Check sheet for the modelled part. Datum: model origin and axes. Units: mm. A direction names the side the tool comes from. Round coordinates to 2 decimals unless told otherwise and drop trailing zeros. Order: outer loops, then holes, each group sorted by start corner. A loop starts at its lowest first (then second) coordinate and runs counter-clockwise, first axis right, second up. Notation, with made-up numbers: (59, 64.5) -> (81, 64.5) arc R6 cw to (81, 70.5) -> close; hole circle Ø3 at (51.25, 70.25). An arc over 180 degrees is marked (long way). Answer in a Markdown table with one row per item.
from build123d import *

# Parameters (mm, degrees)
F1_DEPTH = 76.2
F2_R     = 6.35
F3_DEPTH = 200.038046
F4_R     = 4.5085
F5_DEPTH = 416.492134


with BuildPart() as f1:
    # F0 (on Front) → F1 (new body)
    with BuildSketch(Plane.XZ):
        Polygon((-31.073093, 120.862948), (-81.866795, 120.063045), (-81.866795, -83.136955), (70.533205, -83.136955), (70.533205, -32.336955), (-31.073093, -32.336955), align=None)
    extrude(amount=F1_DEPTH)

    # F2 (on Right) → F3 (cut)
    with BuildSketch(Plane.YZ):
        with Locations((-38.1, 44.662948)):
            Circle(F2_R)
    extrude(amount=-F3_DEPTH, mode=Mode.SUBTRACT)

    # F4 (on Top) → F5 (cut)
    with BuildSketch(Plane.XY):
        with Locations((19.733205, -38.1)):
            Circle(F4_R)
    extrude(amount=-F5_DEPTH, mode=Mode.SUBTRACT)


solid = f1.part
Item 1: Depth check by flat-ended pin: P1, Ø1.5, axis at x = 38, y = -65.5, coming from the +Z side; P2, Ø1, axis at y = -11, z = -25, coming from the +X side. Enter the tip coordinate at first touch or a pass-through.
Result sheet:
| item | result |
|---|---|
| P1 | stops at z = -32.34 |
| P2 | stops at x = -31.07 |
Item 2: Cross-section at D-D (y = -14.5). Record the boundary of the cut face in (x, z).
Result sheet:
| item | result |
|---|---|
| outline | (-81.87, -83.14) -> (70.53, -83.14) -> (70.53, -32.34) -> (-31.07, -32.34) -> (-31.07, 120.86) -> (-81.87, 120.06) -> close |
Item 3: Scan lines: line 1 (X direction, y = -38, z = -60); line 2 (X direction, y = -59, z = 27.5); line 3 (Z direction, x = -28.5, y = -48). Record each from-to range of solid material in increasing order. Write a range as [from, to].
Result sheet:
| item | result |
|---|---|
| line 1 | x = [-81.87, 15.23], [24.24, 70.53] |
| line 2 | x = [-81.87, -31.07] |
| line 3 | z = [-83.14, -32.34] |
Item 4: Cross-section at A-A (y = -38.1). Record the boundary of the cut face in (x, z), and give its area (3 significant figures).
Result sheet:
| item | result |
|---|---|
| outline | (-81.87, -83.14) -> (15.22, -83.14) -> (15.22, -32.34) -> (-31.07, -32.34) -> (-31.07, 38.31) -> (-81.87, 38.31) -> close; (-81.87, 51.01) -> (-31.07, 51.01) -> (-31.07, 120.86) -> (-81.87, 120.06) -> close; (24.24, -83.14) -> (70.53, -83.14) -> (70.53, -32.34) -> (24.24, -32.34) -> close |
| area | 14,400 mm^2 |
Item 5: Set-up check for faces 1 (the flat face through (20, -46, -32.337)), 2 (the flat face through (-41, 0, -2)): record each of +Z, -Z, +X, -X, +Y, -Y from which the full face is reachable in a straight line by a thin tool's end or side.
Result sheet:
| item | result |
|---|---|
| face 1 | +Z, +X, +Y, -Y |
| face 2 | +Z, -Z, +X, -X, +Y |
Item 6: Cross-section at B-B (x = 22). Record the boundary of the cut face in (y, z).
Result sheet:
| item | result |
|---|---|
| outline | (-76.2, -83.14) -> (-42, -83.14) -> (-42, -32.34) -> (-76.2, -32.34) -> close; (-34.2, -83.14) -> (0, -83.14) -> (0, -32.34) -> (-34.2, -32.34) -> close |
Item 7: Mould release check, pull along X, two halves, no side actions. Record for faces 3 (the flat face through (-81.867, -38, 20)), 4 (the flat face through (70.533, -38, -58)), 5 (the cylindrical face through (24.034, -36.746, -57.381)): pulls with the +X half, pulls with the -X half, needs draft (parallel to the pull), parting line crosses it, or undercut.
Result sheet:
| item | result |
|---|---|
| face 3 | pulls with the -X half |
| face 4 | pulls with the +X half |
| face 5 | undercut |
Item 8: Cross-section at C-C (z = 71.5). Record the boundary of the cut face in (x, y), and give its area (3 significant figures).
Result sheet:
| item | result |
|---|---|
| outline | (-81.87, -76.2) -> (-31.07, -76.2) -> (-31.07, 0) -> (-81.87, 0) -> close |
| area | 3,870 mm^2 |
